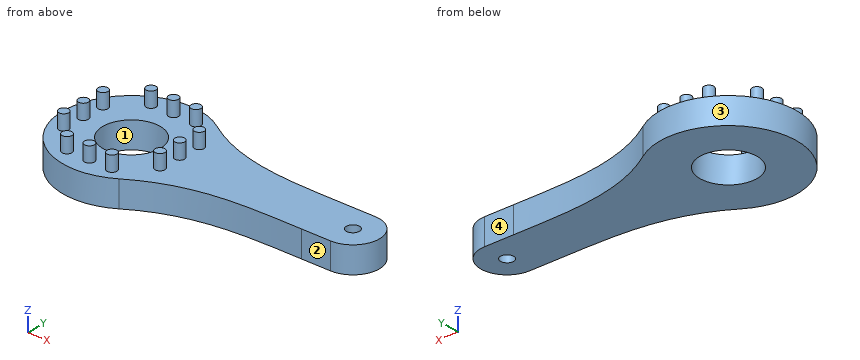
from build123d import *

# Parameters (mm, degrees)
SKETCH1_R           = 4.35
SKETCH1_R_2         = 1
BOSS_EXTRUDE1_DEPTH = 4
SKETCH2_R           = 0.75
BOSS_EXTRUDE2_DEPTH = 2.3


with BuildPart() as part:
    # Sketch1 → Boss-Extrude1 (new body)
    with BuildSketch(Plane.XY):
        with BuildLine():
            Line((30, 4), (34.5, 4))
            ThreePointArc((34.5, 4), (38.5, 0), (34.5, -4))
            Line((34.5, -4), (30, -4))
            add(Edge.make_bspline(
                [(5.686193022, -8.707882), (13.410427979, -3.664004406), (21.266865382, -4), (30, -4)],
                knots=[0, 0, 0, 0, 1, 1, 1, 1], degree=3))
            ThreePointArc((5.686193022, -8.707882), (-10.4, 0), (5.686193022, 8.707882))
            add(Edge.make_bspline(
                [(5.686193022, 8.707882), (13.410427979, 3.664004406), (21.266865382, 4), (30, 4)],
                knots=[0, 0, 0, 0, 1, 1, 1, 1], degree=3))
        make_face()
        Circle(SKETCH1_R, mode=Mode.SUBTRACT)
        with Locations((34.5, 0)):
            Circle(SKETCH1_R_2, mode=Mode.SUBTRACT)
    extrude(amount=BOSS_EXTRUDE1_DEPTH)

    # Sketch2 → Boss-Extrude2 (add)
    with BuildSketch(Plane.XY.offset(4)):
        with Locations(Location((0, 7.5, 0), (0, 0, 180))):
            Circle(SKETCH2_R)
        with Locations(Location((3.5, 7.5, 0), (0, 0, 180))):
            Circle(SKETCH2_R)
        with Locations(Location((-3.5, 7.5, 0), (0, 0, 180))):
            Circle(SKETCH2_R)
        with Locations(Location((3.5, -7.5, 0), (0, 0, 180))):
            Circle(SKETCH2_R)
        with Locations(Location((0, -7.5, 0), (0, 0, 180))):
            Circle(SKETCH2_R)
        with Locations(Location((-3.5, -7.5, 0), (0, 0, 180))):
            Circle(SKETCH2_R)
        with Locations(Location((7.5, 0, 0), (0, 0, 180))):
            Circle(SKETCH2_R)
        with Locations(Location((7.5, 3.5, 0), (0, 0, 180))):
            Circle(SKETCH2_R)
        with Locations(Location((7.5, -3.5, 0), (0, 0, 180))):
            Circle(SKETCH2_R)
        with Locations(Location((-7.5, -3.5, 0), (0, 0, 180))):
            Circle(SKETCH2_R)
        with Locations(Location((-7.5, 0, 0), (0, 0, 180))):
            Circle(SKETCH2_R)
        with Locations(Location((-7.5, 3.5, 0), (0, 0, 180))):
            Circle(SKETCH2_R)
    extrude(amount=BOSS_EXTRUDE2_DEPTH)


solid = part.part
Work out the finished part from the listing and answer in its coordinate system (mm). Face numbers are marked on the shaded views. Coordinates: 2 decimals unless noted, no trailing zeros. Loops run counter-clockwise (first coordinate to the right, second up) from the corner with the lowest first, then second, coordinate; pieces in that order, holes last. Notation, with made-up numbers: (-11.5, 20.5) -> (24.5, 20.5) arc R24 cw to (24.5, 30.5) -> close; hole circle Ø2 at (40.25, -1). An arc over 180 degrees is marked (long way). Write each question's results on one line, items separated by ' | '. Start each with the question number.
1) Find section B-B on z = 5.5. Count the separate pieces of the cut face and the enclosed holes in it, then the cut area to 3 significant figures.
2) Find section C-C on y = 0. Determine the outline of the cut face in (x, z), then the cut area to 3 significant figures.
3) Consider line 1 along Y through (x, z) = (0, 1.95); line 2 along Y through (x, z) = (34.5, 1.65); line 3 along Z through (x, y) = (34, -3.25). Determine where each line is inside the solid, lowest interval first.
4) The mould has two halves that part along Y. Classify the marked faces 1, 2, 3 and 4: pulls with the +Y half, pulls with the -Y half, needs draft (parallel to the pull), parting line crosses it, or undercut.
5) Find section A-A on x = 0. Determine the outline of the cut face in (y, z).
6) Flat-ended cylindrical pins translate along their axes: P1, Ø3, axis at x = 33.5, z = 2.5, coming from the +Y side; P2, Ø7, axis at x = 0, y = 0, coming from the -Z side; P3, Ø10.5, axis at x = 8.5, y = 2, coming from the +Z side; P4, Ø2, axis at y = -4, z = 4, coming from the -X side. Find the tip coordinate at first contact, or state that the pin passes through.
Response values:
1) separate pieces: 12 | enclosed holes: 0 | area: 21.2 mm^2
2) outline: (-10.4, 0) -> (-4.35, 0) -> (-4.35, 4) -> (-6.75, 4) -> (-6.75, 6.3) -> (-8.25, 6.3) -> (-8.25, 4) -> (-10.4, 4) -> close; (4.35, 0) -> (33.5, 0) -> (33.5, 4) -> (8.25, 4) -> (8.25, 6.3) -> (6.75, 6.3) -> (6.75, 4) -> (4.35, 4) -> close; (35.5, 0) -> (38.5, 0) -> (38.5, 4) -> (35.5, 4) -> close | area: 160 mm^2
3) line 1: y = -10.4 to -4.35, 4.35 to 10.4 | line 2: y = -4 to -1, 1 to 4 | line 3: z = 0 to 4
4) face 1: undercut | face 2: pulls with the -Y half | face 3: parting line crosses it | face 4: pulls with the +Y half
5) outline: (-10.4, 0) -> (-4.35, 0) -> (-4.35, 4) -> (-6.75, 4) -> (-6.75, 6.3) -> (-8.25, 6.3) -> (-8.25, 4) -> (-10.4, 4) -> close; (4.35, 0) -> (10.4, 0) -> (10.4, 4) -> (8.25, 4) -> (8.25, 6.3) -> (6.75, 6.3) -> (6.75, 4) -> (4.35, 4) -> close
6) P1: stops at y = 4 | P2: passes through | P3: stops at z = 6.3 | P4: stops at x = -9.96
